```python
from build123d import *

# Parameters (mm, degrees)
BOSS_EXTRUDE1_DEPTH = 3.95
SKETCH2_R           = 3.575
CUT_EXTRUDE1_DEPTH  = 3.95
BOSS_EXTRUDE2_DEPTH = 1.64
SKETCH4_R           = 3.25
CUT_EXTRUDE2_DEPTH  = 63.643819328
CAVITY1_OUTLINE_R   = 3.25
CAVITY1_DEPTH       = 5.59
CAVITY1_START       = 3.19
CAVITY1_2_DEPTH     = 2.4
CUT_EXTRUDE4_DEPTH  = 63.643819328
CUT_EXTRUDE5_START  = -10
SKETCH6_R           = 1
CUT_EXTRUDE5_DEPTH  = 10


# Read off the part's stored shape, not the designer's step: Cavity1
with BuildPart() as part:
    # Sketch1 → Boss-Extrude1 (new body)
    with BuildSketch(Plane(origin=(0, 0, 0), x_dir=(1, 0, 0), z_dir=(0, 1, 0))):
        with BuildLine():
            Line((0, 7), (55, 7))
            ThreePointArc((55, 7), (62, 0), (55, -7))
            Line((55, -7), (0, -7))
            ThreePointArc((0, -7), (-7, 0), (0, 7))
        make_face()
    extrude(amount=BOSS_EXTRUDE1_DEPTH)

    # Sketch2 → Cut-Extrude1 (cut)
    with BuildSketch(Plane.XZ):
        with Locations(Location((0, 0, 0), (0, 0, 270))):
            Circle(SKETCH2_R)
    extrude(amount=-CUT_EXTRUDE1_DEPTH, mode=Mode.SUBTRACT)

    # Sketch3 → Boss-Extrude2 (add)
    with BuildSketch(Plane(origin=(0, 3.95, 0), x_dir=(1, 0, 0), z_dir=(0, 1, 0))):
        with BuildLine():
            Line((0, -7), (55, -7))
            ThreePointArc((55, -7), (62, 0), (55, 7))
            Line((55, 7), (0, 7))
            ThreePointArc((0, 7), (-7, 0), (0, -7))
        make_face()
        with BuildLine():
            Line((13.979308982, 2.569996388), (1.997926282, 3.167540934))
            ThreePointArc((1.997926282, 3.167540934), (-3.745, 0), (1.997926282, -3.167540934))
            Line((1.997926282, -3.167540934), (13.979308982, -2.569996388))
            ThreePointArc((13.979308982, -2.569996388), (16.545, 0), (13.979308982, 2.569996388))
        make_face(mode=Mode.SUBTRACT)
    extrude(amount=BOSS_EXTRUDE2_DEPTH)

    # Sketch4 → Cut-Extrude2 (cut, through all)
    with BuildSketch(Plane(origin=(0, 5.59, 0), x_dir=(1, 0, 0), z_dir=(0, 1, 0))):
        with Locations(Location((55, 0, 0), (0, 0, 270))):
            Circle(SKETCH4_R)
    extrude(amount=-CUT_EXTRUDE2_DEPTH, mode=Mode.SUBTRACT)

    # Cavity1 outline → Cavity1 (cut)
    with BuildSketch(Plane(origin=(0, 0, 0), x_dir=(1, 0, 0), z_dir=(0, 1, 0))):
        with BuildLine():
            Line((58.605551275, 6), (38, 6))
            Line((38, 6), (38, -6))
            Line((38, -6), (58.605551275, -6))
            ThreePointArc((58.605551275, -6), (59.949747468, -4.949747468), (61, -3.605551275))
            Line((61, -3.605551275), (61, 3.605551275))
            ThreePointArc((61, 3.605551275), (59.949747468, 4.949747468), (58.605551275, 6))
        make_face()
        with Locations((55, 0)):
            Circle(CAVITY1_OUTLINE_R, mode=Mode.SUBTRACT)
    extrude(amount=CAVITY1_DEPTH, mode=Mode.SUBTRACT)

    # Cavity1 2 outline → Cavity1 2 (cut)
    with BuildSketch(Plane(origin=(0, 0, 0), x_dir=(1, 0, 0), z_dir=(0, 1, 0)).offset(CAVITY1_START)):
        with BuildLine():
            Line((33.3, 0.5), (34.605619966, 0.5))
            ThreePointArc((34.605619966, 0.5), (36.47164537, 0), (34.605619966, -0.5))
            Line((34.605619966, -0.5), (33.3, -0.5))
            Line((33.3, -0.5), (33.3, -6))
            Line((33.3, -6), (38, -6))
            Line((38, -6), (38, 6))
            Line((38, 6), (33.3, 6))
            Line((33.3, 6), (33.3, 0.5))
        make_face()
        with BuildLine():
            ThreePointArc((61, -3.605551275), (62, 0), (61, 3.605551275))
            Line((61, 3.605551275), (61, -3.605551275))
        make_face()
    extrude(amount=CAVITY1_2_DEPTH, mode=Mode.SUBTRACT)

    # Sketch5 → Cut-Extrude4 (cut, through all)
    with BuildSketch(Plane.XZ):
        with BuildLine():
            Line((61, 3.605551275), (61, -3.605551275))
            ThreePointArc((61, -3.605551275), (62, 0), (61, 3.605551275))
        make_face()
    extrude(amount=-CUT_EXTRUDE4_DEPTH, mode=Mode.SUBTRACT)

    # Sketch6 → Cut-Extrude5 (cut)
    with BuildSketch(Plane(origin=(0, 5.59, 0), x_dir=(1, 0, 0), z_dir=(0, 1, 0)).offset(CUT_EXTRUDE5_START)):
        with Locations(Location((35.47164537, 0, 0), (0, 0, 270))):
            Circle(SKETCH6_R)
    extrude(amount=CUT_EXTRUDE5_DEPTH, mode=Mode.SUBTRACT)


solid = part.part
```
Design review of the part built by this model. Coordinates are the model's own, in mm. A direction names the side the tool comes from. Round coordinates to 2 decimals unless told otherwise and drop trailing zeros. Write each loop counter-clockwise with the first axis right and the second up, starting at its lowest first coordinate (ties: lowest second). Pieces come first, ordered by that corner, then holes.
Item 1: For probe 1 along X at (y, z) = (2.6, 0) (3 decimals); probe 2 along Z at (x, y) = (0, 5.25) (3 decimals); probe 3 along Y at (x, z) = (3.5, -2.25), list the stretches that pass through material, from the lowest coordinate up.
Item 2: We need section B-B on x = 13. Write out the cut boundary in (y, z), and give its area (3 significant figures).
Item 3: We need section C-C on y = 1.2. Write out the cut boundary in (x, z) (3 decimals), and give its area (3 significant figures).
Item 4: For faces 1 (the flat face through (34, 4, -0.5)), 2 (the cylindrical face through (3.545, 1.947, 0.465)), 3 (the flat face through (38, 2, 0)), 4 (the cylindrical face through (-3.743, 4.759, -0.112)), list the 3-axis set-ups (+Z, -Z, +X, -X, +Y, -Y) from which the entire face can be reached by the end or side of a thin tool; tool diameter is ignored.
Item 5: We need section A-A on x = 45. Write out the cut boundary in (y, z).
Item 6: The part is to be moulded in two halves that separate along Z. For faces 5 (the flat face through (27, 3, 7)), 6 (the flat face through (7.905, 4.759, 2.873)), 7 (the flat face through (19, 0, 0)), say which applies: +Z half, -Z half, draft (parallel to the pull), parting line (faces both ways), or undercut.
Item 7: We need section D-D on z = 5. Write out the cut boundary in (x, y).
Item 8: Clearance check with flat-ended pins moving along their axes: pin 1 Ø1.6 at (x, z) = (35.47, 0) entering from +Y; pin 2 Ø2.5 at (y, z) = (1, 0) entering from +X; pin 3 Ø4 at (x, z) = (36.5, -1.5) entering from +Y; pin 4 Ø2 at (y, z) = (5, 2.5) entering from -X. State where each tip first meets the part, or that it passes through.
Returned:
1. probe 1: x = -7 to -3.575, 3.575 to 34.472, 36.472 to 38
1. probe 2: z = -7 to -3.745, 3.745 to 7
1. probe 3: y = 0 to 3.95
2. outline: (0, -7) - (5.59, -7) - (5.59, -2.62) - (3.95, -2.62) - (3.95, 2.62) - (5.59, 2.62) - (5.59, 7) - (0, 7) - close
2. area: 69.7 mm2
3. outline: (0, -7) - (55, -7) arc R7 ccw to (58.606, -6) - (38, -6) - (38, 6) - (58.606, 6) arc R7 ccw to (55, 7) - (0, 7) arc R7 ccw to start; hole circle Ø7.15 at (0, 0); hole circle Ø2 at (35.472, 0)
3. area: 605 mm2
4. face 1: +X, +Y
4. face 2: +Y, -Y
4. face 3: +X, +Y, -Y
4. face 4: +Y
5. outline: (0, -7) - (5.59, -7) - (5.59, -6) - (0, -6) - close; (0, 6) - (5.59, 6) - (5.59, 7) - (0, 7) - close
6. face 5: +Z half
6. face 6: undercut
6. face 7: draft
7. outline: (-4.9, 0) - (38, 0) - (38, 3.19) - (33.3, 3.19) - (33.3, 5.59) - (-4.9, 5.59) - close
8. pin 1: passes through
8. pin 2: stops at x = 38
8. pin 3: stops at y = 3.19
8. pin 4: stops at x = -6.84
